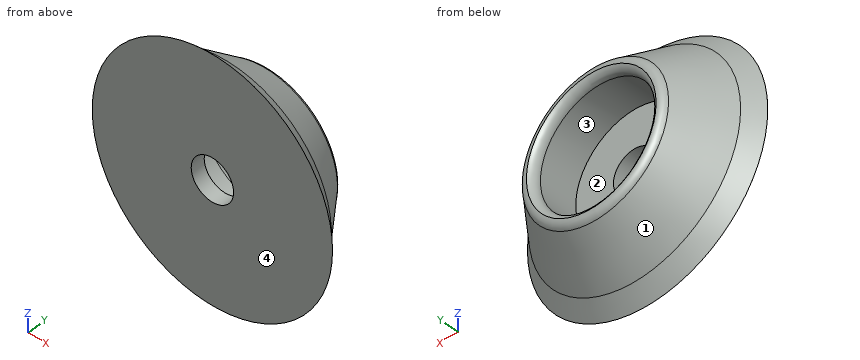
Autodesk Inventor part; units mm, degrees
ref_plane "YZ Plane" through (0, 0, 0) normal (1, 0, 0) x (0, 1, 0)
ref_plane "XZ Plane" through (0, 0, 0) normal (0, 1, 0) x (-1, 0, 0)
ref_plane "XY Plane" through (0, 0, 0) normal (0, 0, 1) x (1, 0, 0)
sketch "Sketch1" plane through (0, 0, 0) normal (0, 1, 0) x (-1, 0, 0)
  circle A0 centre (0, 0) radius 12.5
  circle A1 centre (0, 0) radius 15.5
  circle A2 centre (0, 0) radius 25.5
  circle A3 centre (0, 0) radius 4.5
  dimension "d0" = 25
  dimension "d1" = 31
  dimension "d2" = 51
  dimension "d3" = 9
extrude "Extrusion1" add sketch "Sketch1" along normal blind 3 contours A0 | A1 | A2
chamfer "Chamfer1" distance 3 angle 45 1 edges at (25.5, 3, 0)
extrude "Extrusion2" add sketch "Sketch1" along normal blind 13 contours A1
chamfer "Chamfer2" distance 7 distance2 9 1 edges at (15.5, 3, 0) measured on face at (-19.7987, 3, -3.0313)
fillet "Fillet1" radius 2 2 edges at (15.5, 13, 0) (12.5, 13, 0)
properties part number "boltCap"
Here's how the part is built. I have some questions about the finished solid (model axes, mm). Face numbers are marked on the shaded views. Give positions to 0.01 mm unless a question says otherwise; leave off trailing zeros. Loops run counter-clockwise (first coordinate to the right, second up) from the corner with the lowest first, then second, coordinate; pieces in that order, holes last. Notation, with made-up numbers: (6.25, 4.25) -> (21.25, 4.25) arc R11 cw to (21.25, 14.25) -> close; hole circle Ø7 at (-22.5, -18). An arc over 180 degrees is marked (long way). Answer as a JSON object with one key per item and string values. Group by question number.
Item 1: Thinking about a two-plate mould opening in X: for the marked faces 1, 2, 3 and 4, which applies, pulls with the +X half, pulls with the -X half, needs draft (parallel to the pull), parting line crosses it, or undercut?
Item 2: Will these pins go through, and if not, where does the flat tip stop? pin 1 (6 mm diameter, centred on x = -14.5, y = 10, fed in from -Z); pin 2 (3 mm diameter, centred on y = 5, z = 10.5, fed in from +X); pin 3 (20 mm diameter, centred on x = 0, z = 0, fed in from +Y); pin 4 (1 mm diameter, centred on x = 20, z = 17, fed in from +Y).
Item 3: Imagine slicing it at C-C on y = 1. Write out the boundary of the cut face in (x, z), then the cut area to 3 significant figures.
Item 4: Imagine slicing it at D-D on y = 10. Write out the boundary of the cut face in (x, z).
Item 5: I need wall thicknesses on L1, parallel to X at y = 11, z = -6; L2, parallel to Y at x = -12, z = -0.5; L3, parallel to X at y = 8, z = 0. Which ranges of each line are inside material? Lowest first, please.
Answer list:
{
 "1": {"face 1": "parting line crosses it", "face 2": "undercut", "face 3": "undercut", "face 4": "needs draft"},
 "2": {"pin 1": "stops at z = -14.04", "pin 2": "stops at x = 19.67", "pin 3": "stops at y = 3", "pin 4": "passes through"},
 "3": {"outline": "circle Ø49 at (0, 0); hole circle Ø9 at (0, 0)", "area": "1,820 mm2"},
 "4": {"outline": "circle Ø34.11 at (0, 0); hole circle Ø25 at (0, 0)"},
 "5": {"L1": "x = -15.13 to -10.97, 10.97 to 15.13", "L2": "y = 0 to 3", "L3": "x = -18.61 to -12.5, 12.5 to 18.61"}
}
